```python
from build123d import *

# Parameters (mm, degrees)
SKETCH1_W           = 76.2
SKETCH1_H           = 88.978
SKETCH1_W_2         = 44.45
SKETCH1_H_2         = 50.8
BOSS_EXTRUDE1_DEPTH = 3.175
FILLET1_R           = 5


# Read off the part's stored shape, not the designer's step: AdvancedHole1
with BuildPart() as part:
    # Sketch1 → Boss-Extrude1 (new body)
    with BuildSketch(Plane(origin=(0, 0, 0), x_dir=(1, 0, 0), z_dir=(0, 1, 0))):
        Rectangle(SKETCH1_W, SKETCH1_H)
        Rectangle(SKETCH1_W_2, SKETCH1_H_2, mode=Mode.SUBTRACT)
    extrude(amount=BOSS_EXTRUDE1_DEPTH)

    # AdvancedHole1 outline → AdvancedHole1 (revolve, cut)
    with BuildSketch(Plane(origin=(12.5, 0, -31.75), x_dir=(1, 0, 0), z_dir=(0, 0, 1))):
        Polygon((4, 3.175), (0, 3.175), (0, 0), (2.25, 0), (2.25, 1.425), align=None)
    advancedhole1 = revolve(axis=Axis((12.5, 0, -31.75), (0, 1, 0)), mode=Mode.SUBTRACT)

    # AdvancedHole1 2 outline → AdvancedHole1 2 (revolve, cut)
    with BuildSketch(Plane(origin=(-12.5, 0, -31.75), x_dir=(1, 0, 0), z_dir=(0, 0, 1))):
        Polygon((4, 3.175), (0, 3.175), (0, 0), (2.25, 0), (2.25, 1.425), align=None)
    advancedhole1_2 = revolve(axis=Axis((-12.5, 0, -31.75), (0, 1, 0)), mode=Mode.SUBTRACT)

    # Mirror1: AdvancedHole1, AdvancedHole1 2 across plane
    add(advancedhole1.mirror(Plane.XY), mode=Mode.SUBTRACT)
    add(advancedhole1_2.mirror(Plane.XY), mode=Mode.SUBTRACT)

    # Fillet1
    fillet1_edges = [part.edges().sort_by_distance(p)[0] for p in [
        (-22.225, 1.5875, -25.4),
        (-22.225, 1.5875, 25.4),
        (22.225, 1.5875, 25.4),
        (22.225, 1.5875, -25.4),
    ]]
    fillet(fillet1_edges, radius=FILLET1_R)


solid = part.part
```
Part model, mm, in its own coordinate system. A direction names the side the tool comes from. Give positions to 0.01 mm unless a question says otherwise; leave off trailing zeros. Loops run counter-clockwise (first coordinate to the right, second up) from the corner with the lowest first, then second, coordinate; pieces in that order, holes last. Notation, with made-up numbers: M 9,16.25 L 27,16.25 A13 ccw 27,30.25 Z; hole C -36.5,-14 d7. An arc over 180 degrees is marked long. Return JSON: item names as keys, results as strings.
1) Saw through at A-A, the plane z = 8.5. List the corners of the cut face in (x, y) (3 decimals).
Calculated:
{"outline": "M -38.1,0 L -22.225,0 L -22.225,3.175 L -38.1,3.175 Z; M 22.225,0 L 38.1,0 L 38.1,3.175 L 22.225,3.175 Z"}
2) Saw through at C-C, the plane z = 31.75. List the corners of the cut face in (x, y) (3 decimals), then the cut area to 3 significant figures.
Calculated:
{"outline": "M -38.1,0 L -14.75,0 L -14.75,1.425 L -16.5,3.175 L -38.1,3.175 Z; M -10.25,0 L 10.25,0 L 10.25,1.425 L 8.5,3.175 L -8.5,3.175 L -10.25,1.425 Z; M 14.75,0 L 38.1,0 L 38.1,3.175 L 16.5,3.175 L 14.75,1.425 Z", "area": "207 mm2"}
3) Saw through at D-D, the plane x = 12.5. List the corners of the cut face in (y, z) (3 decimals).
Calculated:
{"outline": "M 0,-44.489 L 3.175,-44.489 L 3.175,-35.75 L 1.425,-34 L 0,-34 Z; M 0,-29.5 L 1.425,-29.5 L 3.175,-27.75 L 3.175,-25.4 L 0,-25.4 Z; M 0,25.4 L 3.175,25.4 L 3.175,27.75 L 1.425,29.5 L 0,29.5 Z; M 0,34 L 1.425,34 L 3.175,35.75 L 3.175,44.489 L 0,44.489 Z"}
4) 3-axis set-ups, long thin cutter, end or side, ignore diameter. For faces 5 (the face through (-11.232, 1.534, -33.74)), 6 (the face through (-22.225, 2, 0)): which of +Z, -Z, +X, -X, +Y, -Y reach the whole face in a straight line?
Calculated:
{"face 5": "+Y", "face 6": "+Y, -Y"}
5) Saw through at B-B, the plane x = -4.5. List the corners of the cut face in (y, z) (3 decimals).
Calculated:
{"outline": "M 0,-44.489 L 3.175,-44.489 L 3.175,-25.4 L 0,-25.4 Z; M 0,25.4 L 3.175,25.4 L 3.175,44.489 L 0,44.489 Z"}
6) Drill centre lines: line 1 (Z direction, x = -12.5, y = 0.6); line 2 (X direction, y = 1.15, z = -31.75); line 3 (Z direction, x = 0, y = 2.4). Where is each one in solid material? Low to high.
Calculated:
{"line 1": "z = -44.49 to -34, -29.5 to -25.4, 25.4 to 29.5, 34 to 44.49", "line 2": "x = -38.1 to -14.75, -10.25 to 10.25, 14.75 to 38.1", "line 3": "z = -44.49 to -25.4, 25.4 to 44.49"}
7) Flat gauge pin, fed straight in: pin 1 Ø3.5 at (x, z) = (-12.5, -31.75) entering from -Y. Where does the tip first touch, or does it go through?
Calculated:
{"pin 1": "passes through"}
8) Pull direction Z, two halves, no side cores. Call faces 1 (the face through (-1, 2, -44.489)), 2 (the face through (-38.1, 2, 1)), 3 (the face through (-1, 2, 44.489)), 4 (the face through (-12.79, 0.72, 33.98)): released by +Z, released by -Z, zero draft, split by the parting line, or undercut.
Calculated:
{"face 1": "released by -Z", "face 2": "zero draft", "face 3": "released by +Z", "face 4": "undercut"}
